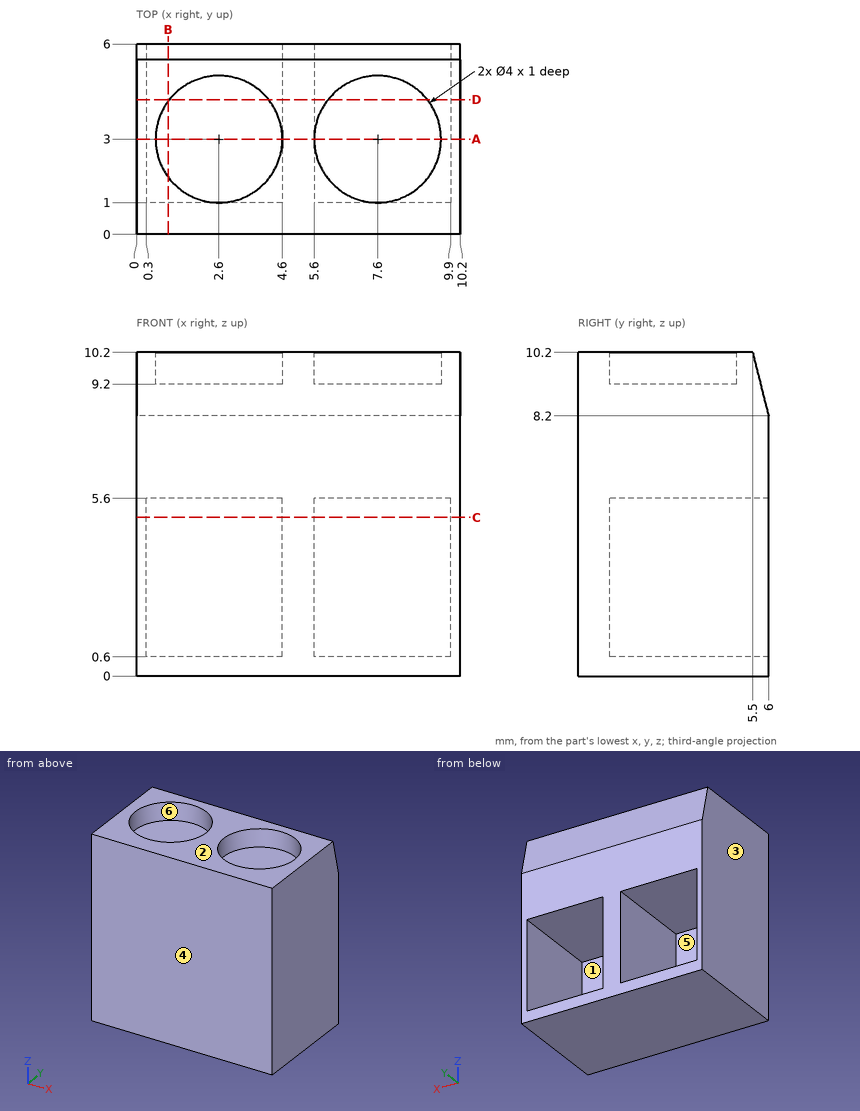
Job drawing, mm, ordinate dimensions from the low corner. One solid piece. A direction names the side the tool comes from. Round coordinates to 2 decimals unless told otherwise and drop trailing zeros. Loops run counter-clockwise (first coordinate to the right, second up) from the corner with the lowest first, then second, coordinate; pieces in that order, holes last. Notation, with made-up numbers: (61, -4.5) -> (72, -4.5) arc R13 cw to (72, 3.5) -> close; hole circle Ø7 at (54, 68.5). An arc over 180 degrees is marked (long way). Use a Markdown table: item, result.
1) Probe line 1 (X direction, y = 4.5, z = 3); line 2 (Z direction, x = 8, y = 2); line 3 (Z direction, x = 9.25, y = 4.25). List the from-to ranges inside material, lowest first. Write a range as [from, to].
The answers:
| item | result |
|---|---|
| line 1 | x = [0, 0.3], [4.6, 5.6], [9.9, 10.2] |
| line 2 | z = [0, 0.6], [5.6, 9.2] |
| line 3 | z = [0, 0.6], [5.6, 10.2] |
2) Cut at A-A, the plane y = 3. List the corners of the cut face in (x, z), and give its area (3 significant figures).
The answers:
| item | result |
|---|---|
| outline | (0, 0) -> (10.2, 0) -> (10.2, 10.2) -> (9.6, 10.2) -> (9.6, 9.2) -> (5.6, 9.2) -> (5.6, 10.2) -> (4.6, 10.2) -> (4.6, 9.2) -> (0.6, 9.2) -> (0.6, 10.2) -> (0, 10.2) -> close; hole (0.3, 0.6) -> (4.6, 0.6) -> (4.6, 5.6) -> (0.3, 5.6) -> close; hole (5.6, 0.6) -> (9.9, 0.6) -> (9.9, 5.6) -> (5.6, 5.6) -> close |
| area | 53.0 mm2 |
3) Cut at B-B, the plane x = 1. List the corners of the cut face in (y, z).
The answers:
| item | result |
|---|---|
| outline | (0, 0) -> (6, 0) -> (6, 0.6) -> (1, 0.6) -> (1, 5.6) -> (6, 5.6) -> (6, 8.2) -> (5.5, 10.2) -> (4.2, 10.2) -> (4.2, 9.2) -> (1.8, 9.2) -> (1.8, 10.2) -> (0, 10.2) -> close |
4) Pull direction X, two halves, no side cores. Call the marked faces 1, 2 and 3: pulls with the +X half, pulls with the -X half, needs draft (parallel to the pull), parting line crosses it, or undercut.
The answers:
| item | result |
|---|---|
| face 1 | undercut |
| face 2 | needs draft |
| face 3 | pulls with the -X half |
5) Cut at C-C, the plane z = 5. List the corners of the cut face in (x, y).
The answers:
| item | result |
|---|---|
| outline | (0, 0) -> (10.2, 0) -> (10.2, 6) -> (9.9, 6) -> (9.9, 1) -> (5.6, 1) -> (5.6, 6) -> (4.6, 6) -> (4.6, 1) -> (0.3, 1) -> (0.3, 6) -> (0, 6) -> close |
6) Tool access for the marked faces 4, 5 and 6: list every direction of +Z, -Z, +X, -X, +Y, -Y with a clear straight run to the whole face (end or side of a thin tool).
The answers:
| item | result |
|---|---|
| face 4 | +Z, -Z, +X, -X, -Y |
| face 5 | +Y |
| face 6 | +Z |
7) Drop a flat-ended pin along its axis: pin 1 Ø1.3 at (x, z) = (8.5, 4) entering from +Y. Give the stop position or say it passes through.
The answers:
| item | result |
|---|---|
| pin 1 | stops at y = 1 |
8) Cut at D-D, the plane y = 4.25. List the corners of the cut face in (x, z).
The answers:
| item | result |
|---|---|
| outline | (0, 0) -> (10.2, 0) -> (10.2, 10.2) -> (9.16, 10.2) -> (9.16, 9.2) -> (6.04, 9.2) -> (6.04, 10.2) -> (4.16, 10.2) -> (4.16, 9.2) -> (1.04, 9.2) -> (1.04, 10.2) -> (0, 10.2) -> close; hole (0.3, 0.6) -> (4.6, 0.6) -> (4.6, 5.6) -> (0.3, 5.6) -> close; hole (5.6, 0.6) -> (9.9, 0.6) -> (9.9, 5.6) -> (5.6, 5.6) -> close |
